Source: CAD feature listing. Evaluate the final solid. Frame: model axes, mm. Face numbers are marked on the shaded views. A direction names the side the tool comes from. Coordinates: 2 decimals unless noted, no trailing zeros. Loops run counter-clockwise (first coordinate to the right, second up) from the corner with the lowest first, then second, coordinate; pieces in that order, holes last.
Item 1: Pin query (flat end, axial travel): pin 1 Ø1 at (x, y) = (4.5, -3) entering from +Z; pin 2 Ø0.6 at (y, z) = (-7.5, 2) entering from +X; pin 3 Ø1 at (y, z) = (-6, 4.5) entering from -X; pin 4 Ø2 at (x, z) = (4, 3) entering from -Y. Return the tip coordinate at first contact, or that it passes through.
Item 2: Line query: probe 1 along Y at (x, z) = (-3, 2); probe 2 along Y at (x, z) = (5.5, 3.25); probe 3 along X at (y, z) = (-6.5, 5). Output: solid intervals per line, ascending.
Item 3: Section query B-B, the plane z = 1. Return the cut outline in (x, y), then the cut area to 3 significant figures.
Item 4: Section query D-D, the plane y = -4. Return the cut outline in (x, z), then the cut area to 3 significant figures.
Item 5: Section query C-C, the plane y = 6.25. Return the cut outline in (x, z).
Item 6: Pull-direction query (Y, two-part tool) for the marked faces 3, 4, 5 and 6; classes: +Y half, -Y half, draft (parallel to the pull), parting line (faces both ways), or undercut.
Item 7: Section query A-A, the plane x = -1.5. Return the cut outline in (y, z).
Item 8: Reachability of the marked faces 1 and 2 from +Z, -Z, +X, -X, +Y, -Y: full face, straight path, thin tool, end or side. Return the list, or none.
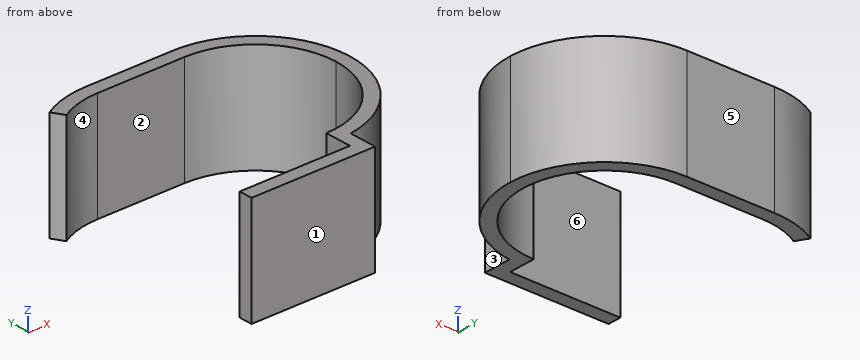
```python
from build123d import *

# Parameters (mm, degrees)
F0_W     = 8.2
F0_H     = 1
F1_DEPTH = 8


with BuildPart() as f1:
    # F0 (on Top) → F1 (new body)
    with BuildSketch(Plane.XY):
        with Locations((-2.6644755177, -7.6461574882)):
            Rectangle(F0_W, F0_H)
        with BuildLine():
            Line((1.4355244823, -6.1461574882), (1.4355244823, -7.1461574882))
            Line((1.4355244823, -7.1461574882), (1.4355244823, -8.1461574882))
            Line((1.4355244823, -8.1461574882), (2.4355244823, -8.1461574882))
            Line((2.4355244823, -8.1461574882), (2.4355244823, -6.0743607185))
            ThreePointArc((2.4355244823, -6.0743607185), (1.9368115199, -6.1281852242), (1.4355244823, -6.1461574882))
        make_face()
        with BuildLine():
            Line((1.4355244823, -5.1461574882), (1.4355244823, -6.1461574882))
            ThreePointArc((1.4355244823, -6.1461574882), (1.9368115199, -6.1281852242), (2.4355244823, -6.0743607185))
            Line((2.4355244823, -6.0743607185), (2.4355244823, -5.1461574882))
            Line((2.4355244823, -5.1461574882), (1.4355244823, -5.1461574882))
        make_face()
        with BuildLine():
            ThreePointArc((7.4355244823, 0.8538425118), (5.6781651694, -3.3887981753), (1.4355244823, -5.1461574882))
            Line((1.4355244823, -5.1461574882), (2.4355244823, -5.1461574882))
            Line((2.4355244823, -5.1461574882), (2.4355244823, -6.0743607185))
            ThreePointArc((2.4355244823, -6.0743607185), (6.7270271044, -3.7287331832), (8.4355244823, 0.8538425118))
            ThreePointArc((8.4355244823, 0.8538425118), (6.3852719506, 5.8035899801), (1.4355244823, 7.8538425118))
            Line((1.4355244823, 7.8538425118), (1.4355244823, 6.8538425118))
            ThreePointArc((1.4355244823, 6.8538425118), (5.6781651694, 5.0964831989), (7.4355244823, 0.8538425118))
        make_face()
        with BuildLine():
            ThreePointArc((-5.0644755177, 7.8538425118), (-6.8762088334, 7.6153232958), (-8.5644755177, 6.9160203383))
            Line((-8.5644755177, 6.9160203383), (-8.0644755177, 6.0499949345))
            ThreePointArc((-8.0644755177, 6.0499949345), (-6.6173897883, 6.6493974695), (-5.0644755177, 6.8538425118))
            Line((-5.0644755177, 6.8538425118), (-5.0644755177, 7.8538425118))
        make_face()
        with BuildLine():
            Line((-1.4589242423, 6.8538425118), (1.4355244823, 6.8538425118))
            Line((1.4355244823, 6.8538425118), (1.4355244823, 7.8538425118))
            ThreePointArc((1.4355244823, 7.8538425118), (-0.2380064128, 7.6508487898), (-1.8144755177, 7.0536408956))
            ThreePointArc((-1.8144755177, 7.0536408956), (-1.6352444565, 6.956331703), (-1.4589242423, 6.8538425118))
        make_face()
        with BuildLine():
            ThreePointArc((-1.8144755177, 7.0536408956), (-3.3909446227, 7.6508487898), (-5.0644755177, 7.8538425118))
            Line((-5.0644755177, 7.8538425118), (-5.0644755177, 6.8538425118))
            Line((-5.0644755177, 6.8538425118), (-2.1700267932, 6.8538425118))
            ThreePointArc((-2.1700267932, 6.8538425118), (-1.9937065789, 6.956331703), (-1.8144755177, 7.0536408956))
        make_face()
        with BuildLine():
            Line((1.4355244823, 7.8538425118), (-5.0644755177, 7.8538425118))
            ThreePointArc((-5.0644755177, 7.8538425118), (-3.3909446227, 7.6508487898), (-1.8144755177, 7.0536408956))
            ThreePointArc((-1.8144755177, 7.0536408956), (-0.2380064128, 7.6508487898), (1.4355244823, 7.8538425118))
        make_face()
        with BuildLine():
            Line((-2.1700267932, 6.8538425118), (-1.4589242423, 6.8538425118))
            ThreePointArc((-1.4589242423, 6.8538425118), (-1.6352444565, 6.956331703), (-1.8144755177, 7.0536408956))
            ThreePointArc((-1.8144755177, 7.0536408956), (-1.9937065789, 6.956331703), (-2.1700267932, 6.8538425118))
        make_face()
    extrude(amount=F1_DEPTH)


solid = f1.part
```
Verdict:
1. pin 1: passes through
1. pin 2: stops at x = 2.44
1. pin 3: stops at x = 1.44
1. pin 4: stops at y = -5.97
2. probe 1: y = -8.15 to -7.15, 6.85 to 7.85
2. probe 2: y = -4.85 to -3.56, 5.27 to 6.55
2. probe 3: x = 1.44 to 2.44
3. outline: (-8.56, 6.92) - (-8.06, 6.05) arc R6 cw to (-5.06, 6.85) - (1.44, 6.85) arc R6 cw to (1.44, -5.15) - (1.44, -7.15) - (-6.76, -7.15) - (-6.76, -8.15) - (2.44, -8.15) - (2.44, -6.07) arc R7 ccw to (1.44, 7.85) - (-5.06, 7.85) arc R7 ccw to start
3. area: 40.5 mm2
4. outline: (4.96, 0) - (6.48, 0) - (6.48, 8) - (4.96, 8) - close
4. area: 12.1 mm2
5. outline: (-8.18, 0) - (-7.69, 0) - (-7.69, 8) - (-8.18, 8) - close; (4.06, 0) - (5.89, 0) - (5.89, 8) - (4.06, 8) - close
6. face 3: draft
6. face 4: undercut
6. face 5: +Y half
6. face 6: undercut
7. outline: (-8.15, 0) - (-7.15, 0) - (-7.15, 8) - (-8.15, 8) - close; (6.85, 0) - (7.85, 0) - (7.85, 8) - (6.85, 8) - close
8. face 1: +Z, -Z, +X, -X, -Y
8. face 2: +Z, -Z
